CAD build for the part. Positions are in the model's coordinates, mm. A direction names the side the tool comes from. Round coordinates to 2 decimals unless told otherwise and drop trailing zeros. Order: outer loops, then holes, each group sorted by start corner. A loop starts at its lowest first (then second) coordinate and runs counter-clockwise, first axis right, second up. Notation, with made-up numbers: (89, 6.25) - (147, 6.25) arc R22 cw to (147, 40.25) - close; hole circle Ø4 at (5.5, -23.75). An arc over 180 degrees is marked (long way). Use one line per item in the form item = value. Start each with the question number.
from build123d import *

# Parameters (mm, degrees)
CROQUIS1_W              = 134
CROQUIS1_H              = 112
SALIENTE_EXTRUIR1_DEPTH = 3
CROQUIS2_W              = 52
CROQUIS2_H              = 92
SALIENTE_EXTRUIR2_DEPTH = 48.812
CORTAR_EXTRUIR1_DEPTH   = 105.902256144
VACIADO1_DEPTH          = 42
CROQUIS4_W              = 52
CROQUIS4_H              = 5
SALIENTE_EXTRUIR3_DEPTH = 90
CROQUIS5_R              = 1.5
CORTAR_EXTRUIR2_DEPTH   = 90
CROQUIS6_R              = 1.5
CORTAR_EXTRUIR3_DEPTH   = 90


# Read off the part's stored shape, not the designer's step: Vaciado1
with BuildPart() as part:
    # Croquis1 → Saliente-Extruir1 (new body)
    with BuildSketch(Plane.XY):
        Rectangle(CROQUIS1_W, CROQUIS1_H)
    extrude(amount=SALIENTE_EXTRUIR1_DEPTH)

    # Croquis2 → Saliente-Extruir2 (add)
    with BuildSketch(Plane.XY.offset(3)):
        with Locations((21, -10)):
            Rectangle(CROQUIS2_W, CROQUIS2_H)
    extrude(amount=SALIENTE_EXTRUIR2_DEPTH)

    # Croquis3 → Cortar-Extruir1 (cut, through all)
    with BuildSketch(Plane.ZY.offset(5)):
        Polygon((51.812, -56), (51.812, 30.154), (44.811949005, 15.153963498), (43.00020398, 16.000146009), (15, -44), (15, -56), align=None)
    extrude(amount=-CORTAR_EXTRUIR1_DEPTH, mode=Mode.SUBTRACT)

    # Vaciado1 outline → Vaciado1 (cut)
    with BuildSketch(Plane.YZ):
        Polygon((-56, 5), (31, 5), (31, 46.812), (19.738299384, 46.812), (20.531058004, 45.114639836), (16.000146009, 43.00020398), (-44, 15), (-56, 15), align=None)
    extrude(amount=VACIADO1_DEPTH, mode=Mode.SUBTRACT)

    # Croquis4 → Saliente-Extruir3 (add)
    with BuildSketch(Plane.XZ.offset(56)):
        with Locations((21, 5.5)):
            Rectangle(CROQUIS4_W, CROQUIS4_H)
    extrude(amount=-SALIENTE_EXTRUIR3_DEPTH)

    # Croquis5 → Cortar-Extruir2 (cut)
    with BuildSketch(Plane.XY.offset(8)):
        with Locations((21, -46)):
            Circle(CROQUIS5_R)
        with Locations((-55, 46)):
            Circle(CROQUIS5_R)
        with Locations((35, 46)):
            Circle(CROQUIS5_R)
    extrude(amount=-CORTAR_EXTRUIR2_DEPTH, mode=Mode.SUBTRACT)

    # Croquis6 → Cortar-Extruir3 (cut)
    with BuildSketch(Plane(origin=(0, 36, 0), x_dir=(1, 0, 0), z_dir=(0, 1, 0))):
        with Locations(Location((30, -31.812, 0), (0, 0, 270))):
            Circle(CROQUIS6_R)
        with Locations(Location((15, -31.812, 0), (0, 0, 270))):
            Circle(CROQUIS6_R)
    extrude(amount=-CORTAR_EXTRUIR3_DEPTH, mode=Mode.SUBTRACT)


solid = part.part
(1) Slice it at A-A (y = -46). Give the cut face in (x, z).
(2) Slice it at D-D (y = 25.5). Give the cut face in (x, z), and give its area (3 significant figures).
(3) Wall check: line 1 (X direction, y = -32.5, z = 15); line 2 (Z direction, x = 15, y = -12.5); line 3 (Z direction, x = -7.5, y = -35). Give the ranges that are in metal, low to high. Write a range as [from, to].
(4) Which spindle directions (+Z, -Z, +X, -X, +Y, -Y) get a long thin tool onto all of the face, cutting with end or side? Do faces 1 (the flat face through (21, 36, 27)), 2 (the cylindrical face through (15.066, 33.535, 30.313)), 3 (the flat face through (21, 25, 46.812)), 4 (the flat face through (-3, -50, 15)), 5 (the flat face through (21, -13, 8)). Say none if no direction does.
(5) Mould opens along X. For faces 6 (the flat face through (42, -3, 23)), 7 (the flat face through (-16, 13, 3)), 8 (the flat face through (-5, 0, 22)) say: pulls with the +X half, pulls with the -X half, needs draft (parallel to the pull), parting line crosses it, or undercut.
(6) Slice it at C-C (x = -55). Give the cut face in (y, z), and give its area (3 significant figures).
(7) Flat gauge pins, fed straight in: P1, Ø2, axis at y = 28, z = 15.5, coming from the -X side; P2, Ø12, axis at x = 19, z = 14.5, coming from the -Y side; P3, Ø5.5, axis at x = 45, y = -52.5, coming from the +Z side. Where does each tip first touch, or does it go through?
(8) Slice it at B-B (x = 21). Give the cut face in (y, z).
Results list:
q1.outline = (-67, 0) - (19.5, 0) - (19.5, 8) - (0, 8) - (0, 15) - (-5, 15) - (-5, 3) - (-67, 3) - close; (22.5, 0) - (67, 0) - (67, 3) - (47, 3) - (47, 15) - (42, 15) - (42, 8) - (22.5, 8) - close
q2.outline = (-67, 0) - (67, 0) - (67, 3) - (47, 3) - (47, 49.64) - (-5, 49.64) - (-5, 3) - (-67, 3) - close; hole (0, 8) - (42, 8) - (42, 46.81) - (0, 46.81) - close
q2.area = 1,200 mm²
q3.line_1 = [-5, 0], [42, 47]
q3.line_2 = [0, 8]
q3.line_3 = [0, 3]
q4.face_1 = +Z, +X, -X, +Y
q4.face_2 = +Y, -Y
q4.face_3 = none
q4.face_4 = +Z, +X, -X, -Y
q4.face_5 = -Y
q5.face_6 = undercut
q5.face_7 = needs draft
q5.face_8 = pulls with the -X half
q6.outline = (-56, 0) - (44.5, 0) - (44.5, 3) - (-56, 3) - close; (47.5, 0) - (56, 0) - (56, 3) - (47.5, 3) - close
q6.area = 327 mm²
q7.P1 = -5
q7.P2 = 31
q7.P3 = 15
q8.outline = (-56, 0) - (-47.5, 0) - (-47.5, 8) - (-56, 8) - close; (-44.5, 0) - (56, 0) - (56, 3) - (36, 3) - (36, 51.81) - (30.15, 51.81) - (15.15, 44.81) - (16, 43) - (20.53, 45.11) - (19.74, 46.81) - (31, 46.81) - (31, 8) - (-44.5, 8) - close
